CAD build for the part. Positions are in the model's coordinates, mm. Coordinates: 2 decimals unless noted, no trailing zeros. Loops run counter-clockwise (first coordinate to the right, second up) from the corner with the lowest first, then second, coordinate; pieces in that order, holes last. Notation, with made-up numbers: (79, 20.5) -> (85, 20.5) arc R26 ccw to (85, 53.5) -> close; hole circle Ø11 at (-35.5, 16). An arc over 180 degrees is marked (long way). Return JSON: item names as keys, results as strings. Group by question number.
(1) Mould opens along Y. For faces 1 (the face through (7.67, 2.41, 12.23)), 2 (the face through (5, 7.84, 12.69)), 3 (the face through (-4.6, 8.3, 1.5)) say: pulls with the +Y half, pulls with the -Y half, needs draft (parallel to the pull), parting line crosses it, or undercut.
(2) Flat gauge pins, fed straight in: pin 1 Ø1 at (y, z) = (-4.5, 9) entering from +X; pin 2 Ø4 at (x, z) = (2.5, 8.5) entering from -Y; pin 3 Ø8 at (x, z) = (4, 3) entering from -Y. Where does each tip first touch, or does it go through?
(3) Saw through at A-A on x = 0. Write the cut outline in (y, z).
(4) Probe L1, parallel to X at y = 0.25, z = 6.5; L2, parallel to Z at x = 0.75, y = -10. List the from-to ranges inside material, lowest first.
(5) Saw through at C-C on z = 8.5. Write the cut outline in (x, y).
```python
from build123d import *

# Parameters (mm, degrees)
F0_R     = 12.3
F0_R_2   = 9.3
F1_DEPTH = 1.5
F0_R_3   = 8.04
F2_DEPTH = 25
F3_SIZE  = 0.8
F4_SIZE  = 0.2


with BuildPart() as f1:
    # F0 (on Top) → F1 (new body)
    with BuildSketch(Plane.XY):
        Circle(F0_R)
        Circle(F0_R_2, mode=Mode.SUBTRACT)
    extrude(amount=F1_DEPTH)

    # F0 (on Top) → F2 (join)
    with BuildSketch(Plane.XY):
        Circle(F0_R_2)
        Circle(F0_R_3, mode=Mode.SUBTRACT)
    extrude(amount=F2_DEPTH)

    # F3
    f3_edges = [f1.edges().sort_by_distance(p)[0] for p in [
        (-9.3, 0, 25),
    ]]
    chamfer(f3_edges, length=F3_SIZE)

    # F4
    f4_edges = [f1.edges().sort_by_distance(p)[0] for p in [
        (-8.04, 0, 25),
    ]]
    chamfer(f4_edges, length=F4_SIZE)


solid = f1.part
```
Geometry results:
{
 "1": {"face 1": "undercut", "face 2": "parting line crosses it", "face 3": "needs draft"},
 "2": {"pin 1": "x = 8.4", "pin 2": "y = -9.29", "pin 3": "y = -12.3"},
 "3": {"outline": "(-12.3, 0) -> (-8.04, 0) -> (-8.04, 24.8) -> (-8.24, 25) -> (-8.5, 25) -> (-9.3, 24.2) -> (-9.3, 1.5) -> (-12.3, 1.5) -> close; (8.04, 0) -> (12.3, 0) -> (12.3, 1.5) -> (9.3, 1.5) -> (9.3, 24.2) -> (8.5, 25) -> (8.24, 25) -> (8.04, 24.8) -> close"},
 "4": {"L1": "-9.3 to -8.04, 8.04 to 9.3", "L2": "0 to 1.5"},
 "5": {"outline": "circle Ø18.6 at (0, 0); hole circle Ø16.08 at (0, 0)"}
}
